Check sheet for the modelled part. Datum: model origin and axes. Units: mm. A direction names the side the tool comes from. Round coordinates to 2 decimals unless told otherwise and drop trailing zeros. Loops run counter-clockwise (first coordinate to the right, second up) from the corner with the lowest first, then second, coordinate; pieces in that order, holes last. Notation, with made-up numbers: (-21, 42) -> (10, 42) arc R33 ccw to (10, 73) -> close; hole circle Ø5 at (4.5, 53.5). An arc over 180 degrees is marked (long way). Use one line per item in the form item = value. Start each with the question number.
(1) Set-up check for faces 1 (the flat face through (-2, -1, 1)), 2 (the flat face through (-1.22, -0.51, -0.86)): record each of +Z, -Z, +X, -X, +Y, -Y from which the full face is reachable in a straight line by a thin tool's end or side.
(2) Sectioned sample at A-A (x = 5). Record the cut outline in (y, z), and give its area (3 significant figures).
(3) Material ranges on probe 1 along X at (y, z) = (-1.05, -1.35); probe 2 along Z at (x, y) = (8, 0.05); probe 3 along X at (y, z) = (2.35, 1.3), recorded low to high. Write a range as [from, to].
(4) Draft check along Y on faces 3 (the cylindrical face through (8.77, -1.5, -0.07)), 4 (the flat face through (0, 2, 0)), 5 (the flat face through (-1, -1, 0)). Enter one of: released by +Y, released by -Y, zero draft, split by the parting line, or undercut.
(5) Go/stop test with a flat-tipped pin: pin 1 (1 mm diameter, centred on x = 9, z = 1.5, fed in from +Y). Record where the tip stops, or that it passes through.
Autodesk Inventor part; units mm, degrees
ref_plane "Work Plane1" through (29, 0, 0) normal (0, -1, 0) x (1, 0, 0)
ref_plane "YZ Plane" through (0, 0, 0) normal (1, 0, 0) x (0, 1, 0)
ref_plane "XZ Plane" through (0, 0, 0) normal (0, 1, 0) x (-1, 0, 0)
sketch "Szkic1" plane through (0, 0, 0) normal (0, 0, 1) x (1, 0, 0)
  line L0 (0.1667, 0) -> (18, 0)
  line L1 (18, 0) -> (18, 1.5)
  line L2 (18, 1.5) -> (1.5, 1.5)
  line L3 (1.5, 1.5) -> (1.1932, 1.5)
  line L4 (1.1932, 1.5) -> (0, 1.5)
  line L5 (0, 1.5) -> (0, 2.75)
  line L6 (0, 2.75) -> (-2, 2.75)
  line L7 (-2, 2.75) -> (-2, 1.1547)
  line L8 (-2, 1.1547) -> (-0.5, 1.1547)
  line L9 (-0.5, 1.1547) -> (0.1667, 0)
  line L10 (-6, 0) -> (22, 0)
  line L11 (0, -0.55) -> (0, 3.3)
  line L12 (1.5, 1.5) -> (0, 1.5) construction
  dimension "d1" = 16.5
  dimension "d2" = 0.3068
  dimension "d3" = 2
  dimension "d4" = 1.5
  dimension "d5" = 60
  dimension "d6" = 3
  dimension "d7" = 3
  dimension "d8" = 2.3094
  dimension "d9" = 5.5
  dimension "d26" = 18
revolve "Bryła" add sketch "Szkic1" angle 360 about axis through (0.1667, 0, 0) along (1, 0, 0) contours L9 L11 L4 L3 L2 L1 L0 | L9 L8 L7 L6 L5 L11
sketch "Szkic2" plane through (-2, 0, 0) normal (-1, 0, 0) x (0, 0, 1)
  circle A0 centre (0, 0) radius 1.1547
  line L0 (0, -3.85) -> (0, 3.85)
  line L1 (-3.85, 0) -> (3.85, 0)
  line L2 (1.1547, 0) -> (0.5774, -1)
  line L3 (0.5774, -1) -> (-0.5774, -1)
  line L4 (-0.5774, -1) -> (-1.1547, 0)
  line L5 (-1.1547, 0) -> (-0.5774, 1)
  line L6 (-0.5774, 1) -> (0.5774, 1)
  line L7 (0.5774, 1) -> (1.1547, 0)
  point P0 (0, 0)
extrude "Szczelina" add sketch "Szkic2" against normal up to next contours L7 A0 | A0 L2 | L6 L0 A0 | A0 L0 L3 | L0 L6 A0 | A0 L3 L0 | L4 A0 | A0 L5
fillet "Zaokrąglenie1" radius 0.3 1 edges at (-2, -2.75, 0)
thread "Gwint"
chamfer "Faza1" distance 0.3067 distance2 0.3067 1 edges at (18, -1.5, 0) measured on face at (18, -0.4645, -0.4115)
ref_plane "Work Plane1" through (29, 0, 0) normal (0, -1, 0) x (1, 0, 0)
fillet "Fillet2" radius 0.1 1 edges at (0, -1.5, 0)
equation "\"d1\" = GEL"
equation "\"d3\" = KOH"
equation "\"d4\" = INTI"
equation "\"d6\" = GD"
equation "\"d7\" = BDM"
equation "\"d8\" = 1.1547 * SW"
equation "\"d9\" = KOD"
equation "\"d26\" = NLG"
equation "\"d30\" = R"
equation "\"d17\" = RR"
equation "\"d13\" = GEL"
equation "\"d15\" = -0.5 * SPD + 0.5 * GD"
equation "\"d16\" = GUL"
equation "\"GD\" = NND"
equation "\"NLG\" = 18"
equation "\"GEL\" = 16.5"
equation "\"KOD\" = 5.5"
equation "\"KOH\" = 2"
equation "\"INTI\" = 1.5"
equation "\"GAL\" = 0.61345 * PTC"
equation "\"GUL\" = 0.61345 * PTC"
equation "\"BDM\" = NND"
equation "\"SW\" = 2"
equation "\"RR\" = 0.3"
equation "\"SPD\" = NND - 1.2269 * PTC"
equation "\"R\" = 0.1"
equation "\"TOA\" = 30deg"
equation "\"GD1\" = THREADDIA - 1.2269 * PTC"
equation "\"THREADDIA\" = 3"
equation "\"FAWI\" = 45deg"
equation "\"ANG\" = 120deg"
equation "\"PTC\" = 0.5"
equation "\"NND\" = 3"
equation "\"E0\" = 1.155 * SW"
properties part number "DIN 7984 - M3 x 18" material "Stal, miękka"
Checks:
q1.face_1 = +Z, -Z, -X, +Y, -Y
q1.face_2 = -X
q2.outline = circle Ø3 at (0, 0)
q2.area = 7.07 mm2
q3.probe_1 = [-2, 0]
q3.probe_2 = [-1.5, 1.5]
q3.probe_3 = [-1.89, 0]
q4.face_3 = split by the parting line
q4.face_4 = zero draft
q4.face_5 = undercut
q5.pin_1 = 1.12
